from build123d import *

# Parameters (mm, degrees)
F1_DEPTH = 63.5
F2_R     = 50.8


with BuildPart() as f1:
    # F0 (on Front) → F1 (new body, symmetric)
    with BuildSketch(Plane.XZ):
        Polygon((140.708246, 22.779214), (-37.091754, 22.779214), (-37.091754, -40.720786), align=None)
    extrude(amount=F1_DEPTH, both=True)

    # F2
    f2_edges = [f1.edges().sort_by_distance(p)[0] for p in [
        (51.808246, 63.5, -8.970786),
        (51.808246, -63.5, -8.970786),
    ]]
    fillet(f2_edges, radius=F2_R)


solid = f1.part
For this review, take the finished solid that the model builds, in its own axes (mm). Give positions to 0.01 mm unless a question says otherwise; leave off trailing zeros. Loops run counter-clockwise (first coordinate to the right, second up) from the corner with the lowest first, then second, coordinate; pieces in that order, holes last.
Item 1: Insertion check: pin 1 (5 mm diameter, centred on x = 69.5, y = -1, fed in from -Z); pin 2 (3 mm diameter, centred on x = 100, y = -34.5, fed in from -Z); pin 3 (1.5 mm diameter, centred on x = 76.5, y = -49, fed in from -Z). Each pin has a flat end and moves straight along its axis. Give the tip position at first contact, or say it passes through.
Item 2: For line 1 along Y through (x, z) = (0, -10.5); line 2 along Y through (x, z) = (-18.5, -12.5); line 3 along Z through (x, y) = (-27.5, 16.5), list the stretches that pass through material, from the lowest coordinate up.
Item 3: Take a section at B-B, the plane y = 32.5. State the section outline as (x, z) points.
Item 4: Take a section at A-A, the plane y = 3. State the section outline as (x, z) points.
Calculated:
1. pin 1: stops at z = -3.55
1. pin 2: stops at z = 12.55
1. pin 3: stops at z = 15.21
2. line 1: y = -49.69 to 49.69
2. line 2: y = -53.34 to 53.34
2. line 3: z = -37.14 to 22.78
3. outline: (-37.09, -36.45) - (128.76, 22.78) - (-37.09, 22.78) - close
4. outline: (-37.09, -40.72) - (140.71, 22.78) - (-37.09, 22.78) - close
